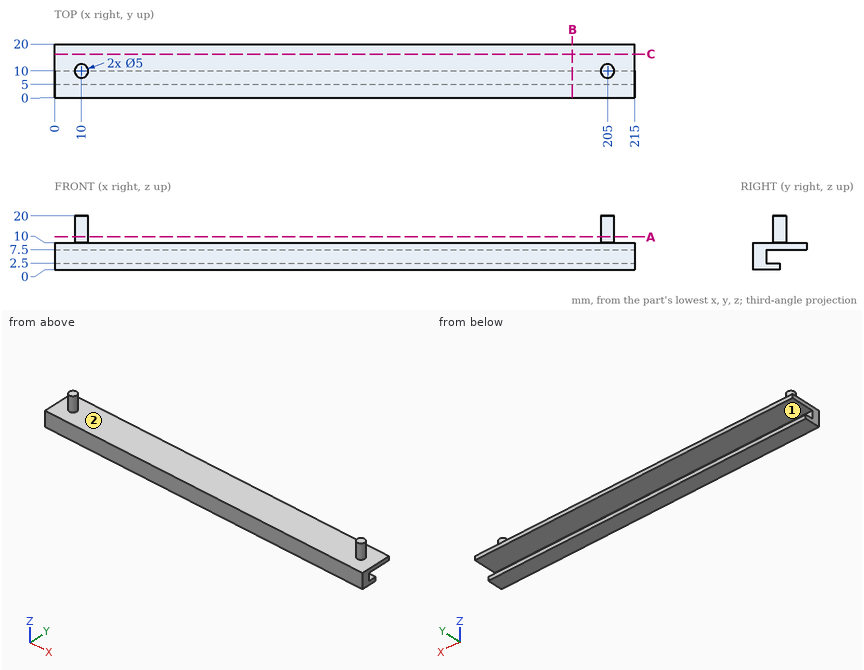
Could you check a few things on this drawing? It's one solid part, dimensions in mm from its lowest x, y, z. Round coordinates to 2 decimals unless told otherwise and drop trailing zeros. Write each loop counter-clockwise with the first axis right and the second up, starting at its lowest first coordinate (ties: lowest second). Pieces come first, ordered by that corner, then holes. Notation, with made-up numbers: M 86.25,-19 L 141.25,-19 A19 ccw 141.25,-4 Z; hole C 28,69 d6. An arc over 180 degrees is marked long. Answer as CSV lines item,"result". Start each with the question number.
1. Suppose I cut it at A-A on z = 12.25. Write out the boundary of the cut face in (x, y).
2. I need wall thicknesses on probe 1 along Z at (x, y) = (161, 9.75); probe 2 along Z at (x, y) = (37, 18.75); probe 3 along Z at (x, y) = (76.5, 1.25). Which ranges of each line are inside material? Lowest first, please.
3. Thinking about a two-plate mould opening in X: for the marked faces 1 and 2, which applies, released by +X, released by -X, zero draft, split by the parting line, or undercut?
4. Suppose I cut it at C-C on y = 16.25. Write out the boundary of the cut face in (x, z), then the cut area to 4 significant figures.
5. I'm going to push flat-ended pins straight in: pin 1 Ø1 at (x, y) = (118, 8.5) entering from +Z; pin 2 Ø7.5 at (x, y) = (111, 15) entering from -Z; pin 3 Ø3 at (y, z) = (8, 8) entering from -X; pin 4 Ø3 at (x, z) = (94, 2) entering from +Y. Where does each tip first touch, or does it pass through?
6. Suppose I cut it at B-B on x = 192. Write out the boundary of the cut face in (y, z), then the cut area to 3 significant figures.
Check result:
1,outline,"C 10,10 d5; C 205,10 d5"
2,probe 1,"z = 0 to 2.5, 7.5 to 10"
2,probe 2,"z = 7.5 to 10"
2,probe 3,"z = 0 to 10"
3,face 1,"zero draft"
3,face 2,"undercut"
4,outline,"M 0,7.5 L 215,7.5 L 215,10 L 0,10 Z"
4,area,"537.5 mm2"
5,pin 1,"stops at z = 10"
5,pin 2,"stops at z = 7.5"
5,pin 3,"stops at x = 0"
5,pin 4,"stops at y = 10"
6,outline,"M 0,0 L 10,0 L 10,2.5 L 5,2.5 L 5,7.5 L 20,7.5 L 20,10 L 0,10 Z"
6,area,"100 mm2"
